```python
from build123d import *

# Parameters (mm, degrees)
ESBO_O1_R                = 32
RESSALTO_EXTRUS_O1_DEPTH = 10
FILETE1_R                = 5
ESBO_O2_R                = 27
CORTE_EXTRUS_O1_DEPTH    = 5


with BuildPart() as part:
    # Esboço1 → Ressalto-extrusão1 (new body)
    with BuildSketch(Plane.XY):
        Circle(ESBO_O1_R)
    extrude(amount=RESSALTO_EXTRUS_O1_DEPTH)

    # Filete1
    filete1_edges = [part.edges().sort_by_distance(p)[0] for p in [
        (-32, 0, 10),
    ]]
    fillet(filete1_edges, radius=FILETE1_R)

    # Esboço2 → Corte-extrusão1 (cut)
    with BuildSketch(Plane(origin=(0, 0, 0), x_dir=(-1, 0, 0), z_dir=(0, 0, -1))):
        Circle(ESBO_O2_R)
    extrude(amount=-CORTE_EXTRUS_O1_DEPTH, mode=Mode.SUBTRACT)


solid = part.part
```
Can you work these out from the model? Positions are in its coordinate system, mm. A direction names the side the tool comes from. Round coordinates to 2 decimals unless told otherwise and drop trailing zeros. Order: outer loops, then holes, each group sorted by start corner. A loop starts at its lowest first (then second) coordinate and runs counter-clockwise, first axis right, second up.
(1) We'd pull the mould along Y, two halves only. Please class faces 3 (the face through (-6.94, -31.24, 2.46)), 4 (the face through (5.85, -26.36, 2.46)), 5 (the face through (-14, -24, 0)): +Y half, -Y half, draft (parallel to the pull), parting line (faces both ways), or undercut.
Results are:
face 3: parting line
face 4: undercut
face 5: draft
(2) On a 3-axis mill with a long thin cutter (end or side, diameter ignored), from which of +Z, -Z, +X, -X, +Y, -Y can I reach the whole of each face in a straight line? I mean faces 1 (the face through (0, 0, 10)), 2 (the face through (0, 0, 5)). Say none if no direction works.
Results are:
face 1: +Z, +X, -X, +Y, -Y
face 2: -Z
(3) If I drill on L1, parallel to Y at x = 0, z = 2.95; L2, parallel to Z at x = -17.5, y = 5.5; L3, parallel to Y at x = 14.5, z = 4, over which ranges is the centre line in solid material (lowest first)?
Results are:
L1: y = -32 to -27, 27 to 32
L2: z = 5 to 10
L3: y = -28.53 to -22.78, 22.78 to 28.53
(4) If we section it at D-D (z = 9): Please give me the cut outline in (x, y), plus the area to 3 significant figures.
Results are:
outline: circle Ø60 at (0, 0)
area: 2,830 mm2
(5) If we section it at A-A (y = 0): Please give me the cut outline in (x, z), plus the area to 3 significant figures.
Results are:
outline: (-32, 0) - (-27, 0) - (-27, 5) - (27, 5) - (27, 0) - (32, 0) - (32, 5) arc R5 ccw to (27, 10) - (-27, 10) arc R5 ccw to (-32, 5) - close
area: 359 mm2
(6) I'm going to push flat-ended pins straight in: pin 1 (8 mm diameter, centred on x = 7, y = -15.5, fed in from -Z); pin 2 (1.5 mm diameter, centred on x = -8, z = 1.5, fed in from +Y); pin 3 (6 mm diameter, centred on y = 21.5, z = 8.5, fed in from +X). Where does each tip first touch, or does it pass through?
Results are:
pin 1: stops at z = 5
pin 2: stops at y = 31.17
pin 3: stops at x = 25.31
(7) If we section it at C-C (z = 1.5): Please give me the cut outline in (x, y).
Results are:
outline: circle Ø64 at (0, 0); hole circle Ø54 at (0, 0)
